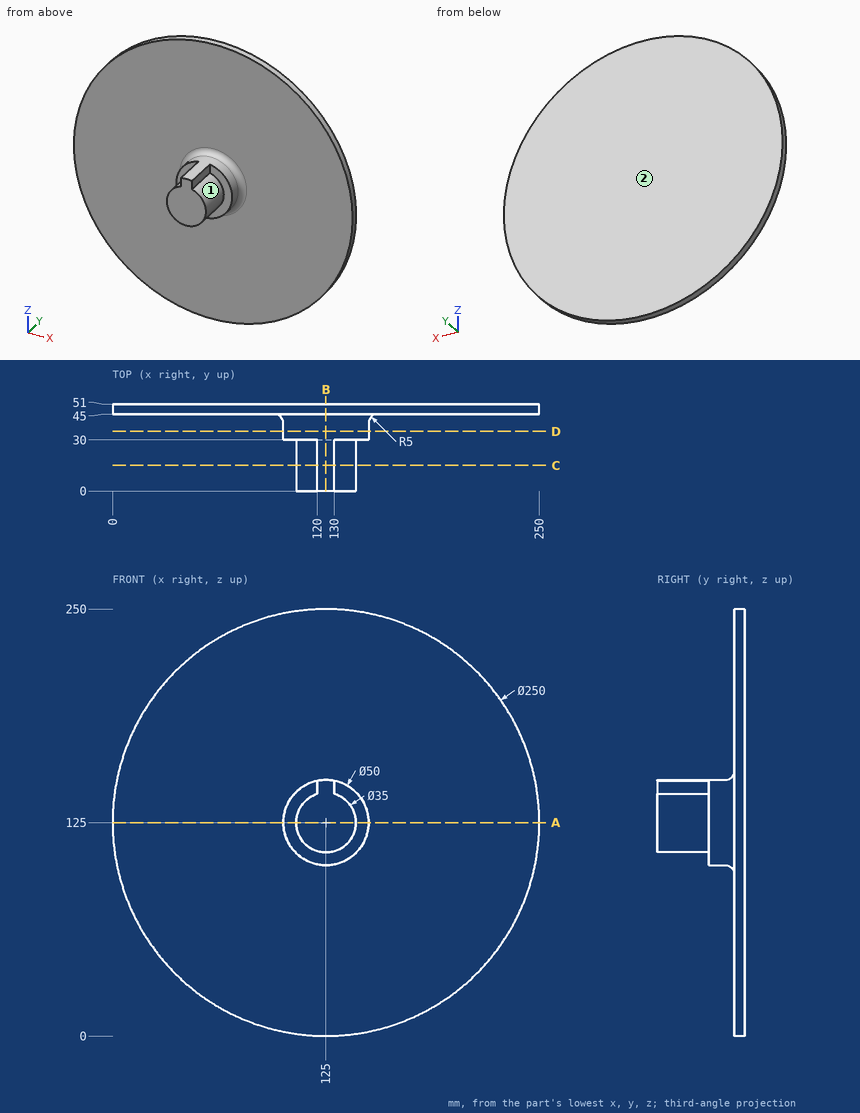
Job drawing, mm, ordinate dimensions from the low corner. One solid piece. A direction names the side the tool comes from. Give positions to 0.01 mm unless a question says otherwise; leave off trailing zeros. Order: outer loops, then holes, each group sorted by start corner. A loop starts at its lowest first (then second) coordinate and runs counter-clockwise, first axis right, second up. Notation, with made-up numbers: M -26.75,17.5 L 32.25,17.5 A32 ccw 32.25,53.5 Z; hole C 38,-10 d4. An arc over 180 degrees is marked long. Put each result on its own line as item: value. Start each with the question number.
(1) Band-saw the part on A-A on z = 125. Give the cut face in (x, y).
(2) Band-saw the part on D-D on y = 35. Give the cut face in (x, z).
(3) Band-saw the part on C-C on y = 15. Give the cut face in (x, z), then the cut area to 3 significant figures.
(4) Tool access for the marked faces 1 and 2: list every direction of +Z, -Z, +X, -X, +Y, -Y with a clear straight run to the whole face (end or side of a thin tool).
(5) Band-saw the part on B-B on x = 125. Give the cut face in (y, z).
(6) Pin check, flat tips, straight feed: pin 1 Ø12 at (x, z) = (221, 52.5) entering from -Y; pin 2 Ø8.5 at (y, z) = (21, 144.5) entering from -X; pin 3 Ø2.5 at (y, z) = (12.5, 144) entering from +X. Stop position of each tip, or through.
(7) Drill centre lines: L1, parallel to Y at x = 199, z = 152; L2, parallel to X at y = 45.5, z = 146.5; L3, parallel to Z at x = 104, y = 35.5. Where is each one in solid material? Low to high. Write a range as [from, to].
Results below:
1. outline: M 0,45 L 95,45 A5 cw 100,40 L 100,30 L 107.5,30 L 107.5,0 L 142.5,0 L 142.5,30 L 150,30 L 150,40 A5 cw 155,45 L 250,45 L 250,51 L 0,51 Z
2. outline: C 125,125 d50
3. outline: M 120,141.77 A17.5 ccw long 130,141.77 L 130,149.49 A25 ccw 120,149.49 Z
3. area: 1,040 mm2
4. face 1: -Y
4. face 2: +Z, -Z, +X, -X, +Y
5. outline: M 0,107.5 L 30,107.5 L 30,100 L 40,100 A5 cw 45,95 L 45,0 L 51,0 L 51,250 L 45,250 L 45,155 A5 cw 40,150 L 0,150 Z
6. pin 1: stops at y = 45
6. pin 2: stops at x = 116.42
6. pin 3: stops at x = 130
7. L1: y = [45, 51]
7. L2: x = [1.86, 248.14]
7. L3: z = [111.44, 138.56]
